Could you check a few things on this model? Use its own coordinates, in mm. Coordinates: 2 decimals unless noted, no trailing zeros. Loops run counter-clockwise (first coordinate to the right, second up) from the corner with the lowest first, then second, coordinate; pieces in that order, holes last. Notation, with made-up numbers: (25.25, -40) -> (82.25, -40) arc R13 ccw to (82.25, -36) -> close; hole circle Ø6 at (4.25, 24). An arc over 180 degrees is marked (long way). One line per question, with ' | ' between items.
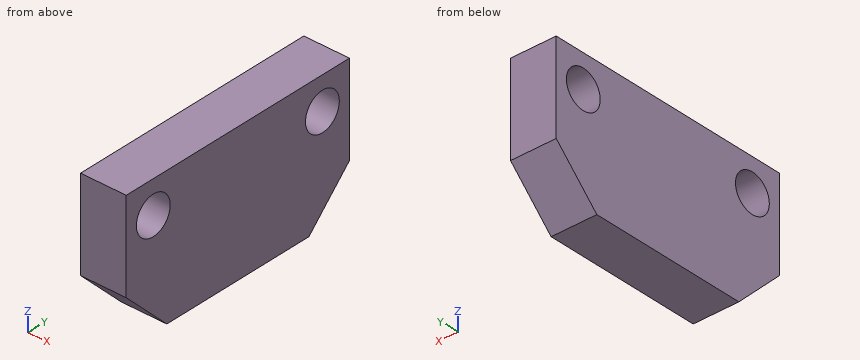
```python
from build123d import *

# Parameters (mm, degrees)
CYLINDER_R              = 2.5
CYLINDER_DEPTH          = 10
CYLINDER_PITCH_ANGLE    = 90
CYLINDER001_R           = 2.5
CYLINDER001_DEPTH       = 10
CYLINDER001_PITCH_ANGLE = 90
BOX_W                   = 6
BOX_H                   = 33
BOX_DEPTH               = 18
CHAMFER_SIZE            = 6


with BuildPart() as cilindro:
    # Cylinder → Cylinder (new body)
    with BuildSketch(Plane.XY):
        Circle(CYLINDER_R)
    extrude(amount=CYLINDER_DEPTH)


with BuildPart() as cilindro_1:
    # Cylinder pitch: moved
    add(cilindro.part.rotate(Axis((0, 0, 0), (0, 1, 0)), CYLINDER_PITCH_ANGLE))


with BuildPart() as cilindro_2:
    # Cylinder placement: moved
    add(cilindro_1.part.moved(Location((28, 7, 61))))


with BuildPart() as fusion:
    # Cylinder001 → Cylinder001 (new body)
    with BuildSketch(Plane.XY):
        Circle(CYLINDER001_R)
    extrude(amount=CYLINDER001_DEPTH)


with BuildPart() as fusion_1:
    # Cylinder001 pitch: moved
    add(fusion.part.rotate(Axis((0, 0, 0), (0, 1, 0)), CYLINDER001_PITCH_ANGLE))


with BuildPart() as fusion_2:
    # Cylinder001 placement: moved
    add(fusion_1.part.moved(Location((28, -18, 61))))

    # Fusion: union Cilindro
    add(cilindro_2.part)


with BuildPart() as soporte_leds:
    # Box → Box (new body)
    with BuildSketch(Plane(origin=(30, -22, 47.3), x_dir=(1, 0, 0), z_dir=(0, 0, 1))):
        with Locations((3, 16.5)):
            Rectangle(BOX_W, BOX_H)
    extrude(amount=BOX_DEPTH)

    # Chamfer
    chamfer_edges = [soporte_leds.edges().sort_by_distance(p)[0] for p in [
        (33, -22, 47.3),
        (33, 11, 47.3),
    ]]
    chamfer(chamfer_edges, length=CHAMFER_SIZE)

    # Cut: cut Fusion
    add(fusion_2.part, mode=Mode.SUBTRACT)


solid = soporte_leds.part
```
Q1. For pin 1 (8 mm diameter, centred on y = -18, z = 61, fed in from -X); pin 2 (4.5 mm diameter, centred on y = 7, z = 61, fed in from +X), each with a flat end and sliding along its axis, tell me the tip position at first contact or that it passes through.
Values follow:
pin 1: stops at x = 30 | pin 2: passes through
Q2. Imagine slicing it at C-C on x = 34.5. Write out the boundary of the cut face in (y, z), plus the area to 3 significant figures.
Values follow:
outline: (-22, 53.3) -> (-16, 47.3) -> (5, 47.3) -> (11, 53.3) -> (11, 65.3) -> (-22, 65.3) -> close; hole circle Ø5 at (-18, 61); hole circle Ø5 at (7, 61) | area: 519 mm2
Q3. Imagine slicing it at A-A on z = 61. Write out the boundary of the cut face in (x, y), plus the area to 3 significant figures.
Values follow:
outline: (30, -22) -> (36, -22) -> (36, -20.5) -> (30, -20.5) -> close; (30, -15.5) -> (36, -15.5) -> (36, 4.5) -> (30, 4.5) -> close; (30, 9.5) -> (36, 9.5) -> (36, 11) -> (30, 11) -> close | area: 138 mm2
Q4. Imagine slicing it at D-D on z = 59. Write out the boundary of the cut face in (x, y), plus the area to 3 significant figures.
Values follow:
outline: (30, -22) -> (36, -22) -> (36, -19.5) -> (30, -19.5) -> close; (30, -16.5) -> (36, -16.5) -> (36, 5.5) -> (30, 5.5) -> close; (30, 8.5) -> (36, 8.5) -> (36, 11) -> (30, 11) -> close | area: 162 mm2
Q5. Please list where these lines run through material, in increasing order: L1, parallel to Y at x = 31.55, z = 61; L2, parallel to Y at x = 34.9, z = 58.75; L3, parallel to Z at x = 31.5, y = -18. Write a range as [from, to].
Values follow:
L1: y = [-22, -20.5], [-15.5, 4.5], [9.5, 11] | L2: y = [-22, -19.09], [-16.91, 5.91], [8.09, 11] | L3: z = [49.3, 58.5], [63.5, 65.3]
Q6. Imagine slicing it at B-B on y = 7. Write out the boundary of the cut face in (x, z), plus the area to 3 significant figures.
Values follow:
outline: (30, 49.3) -> (36, 49.3) -> (36, 58.5) -> (30, 58.5) -> close; (30, 63.5) -> (36, 63.5) -> (36, 65.3) -> (30, 65.3) -> close | area: 66.0 mm2
